Read the model definition and answer for the solid it produces. Units are mm, in the model's axes. A direction names the side the tool comes from. Coordinates: 2 decimals unless noted, no trailing zeros. Write each loop counter-clockwise with the first axis right and the second up, starting at its lowest first coordinate (ties: lowest second). Pieces come first, ordered by that corner, then holes.
(1) Which of the six approach directions +Z, -Z, +X, -X, +Y, -Y give full straight-line access (tool end or side, diameter ignored) to faces 1 (the flat face through (0, -50.5, -13)), 2 (the flat face through (0, -15, -13)), 3 (the cylindrical face through (-7.509, -2.535, 23.846))?
(2) Find the intervals of material crossed by probe 1 along X at (y, z) = (-60, 0) (3 decimals); probe 2 along Y at (x, z) = (22.5, 8.5); probe 3 along X at (y, z) = (-59, 11.5), in increasing order.
(3) Section C-C on x = -5.5 is taken. Write down the section's boundary in (y, z), then the cut area to 3 significant figures.
(4) Given pin 1 (5 mm diameter, centred on x = 0, z = -13.125, fed in from -Y); pin 2 (3 mm diameter, centred on x = 14, z = -0.5, fed in from +Y); pin 3 (8 mm diameter, centred on x = -5, y = -27.5, fed in from +Z), each flat-ended and moving along its own axis, determine where each tip first touches the part or whether it passes through.
(5) Section D-D on y = -39.5 is taken. Write down the section's boundary in (x, z).
(6) Section B-B on y = -58.5 is taken. Write down the section's boundary in (x, z) (3 decimals), then the cut area to 3 significant figures.
from build123d import *

# Parameters (mm, degrees)
SKIZZE5_R                       = 2.8
SCHNITT_LINEAR_AUSTRAGEN1_DEPTH = 15
SCHNITT_LINEAR_START            = -15
SKIZZE7_R                       = 2.8
SCHNITT_LINEAR_AUSTRAGEN2_DEPTH = 15


with BuildPart() as part:
    # Skizze4 → Rotation1 (revolve)
    with BuildSketch(Plane(origin=(0, 0, 0), x_dir=(0, 0, -1), z_dir=(1, 0, 0)), mode=Mode.PRIVATE) as rotation1_sk:
        Polygon((8.75, 0), (25, 0), (25, -5), (19.5, -5), (19.5, -6), (17.5, -6), (17.5, -65.5), (8.75, -65.5), align=None)
    revolve(rotation1_sk.sketch.rotate(Axis((0, 0, 0), (0, -1, 0)), 180), axis=Axis((0, 0, 0), (0, -1, 0)))

    # Skizze5 → Schnitt-Linear austragen1 (cut)
    with BuildSketch(Plane(origin=(0, 0, 0), x_dir=(1, 0, 0), z_dir=(0, 1, 0))):
        with Locations(Location((0, 13.125, 0), (0, 0, 270))):
            Circle(SKIZZE5_R)
        with Locations(Location((13.125, 0, 0), (0, 0, 270))):
            Circle(SKIZZE5_R)
        with Locations(Location((0, -13.125, 0), (0, 0, 270))):
            Circle(SKIZZE5_R)
        with Locations(Location((-13.125, 0, 0), (0, 0, 270))):
            Circle(SKIZZE5_R)
    extrude(amount=-SCHNITT_LINEAR_AUSTRAGEN1_DEPTH, mode=Mode.SUBTRACT)

    # Skizze7 → Schnitt-Linear austragen2 (cut)
    with BuildSketch(Plane.XZ.offset(65.5).offset(SCHNITT_LINEAR_START)):
        with Locations(Location((13.125, 0, 0), (0, 0, 90))):
            Circle(SKIZZE7_R)
        with Locations(Location((0, -13.125, 0), (0, 0, 90))):
            Circle(SKIZZE7_R)
        with Locations(Location((-13.125, 0, 0), (0, 0, 90))):
            Circle(SKIZZE7_R)
        with BuildLine():
            ThreePointArc((0, 15.925), (-2.8, 13.125), (0, 10.325))
            Line((0, 10.325), (0, 15.925))
        make_face()
        with BuildLine():
            Line((0, 15.925), (0, 10.325))
            ThreePointArc((0, 10.325), (1.979898987, 11.145101013), (2.8, 13.125))
            ThreePointArc((2.8, 13.125), (1.979898987, 15.104898987), (0, 15.925))
        make_face()
    extrude(amount=SCHNITT_LINEAR_AUSTRAGEN2_DEPTH, mode=Mode.SUBTRACT)


solid = part.part
Response:
1. face 1: -Y
1. face 2: +Y
1. face 3: +Y, -Y
2. probe 1: x = -17.5 to -15.925, -10.325 to -8.75, 8.75 to 10.325, 15.925 to 17.5
2. probe 2: y = -5 to 0
2. probe 3: x = -13.19 to -2.28, 2.28 to 13.19
3. outline: (-65.5, -16.61) - (-6, -16.61) - (-6, -18.71) - (-5, -18.71) - (-5, -24.39) - (0, -24.39) - (0, -6.81) - (-65.5, -6.81) - close; (-65.5, 6.81) - (0, 6.81) - (0, 24.39) - (-5, 24.39) - (-5, 18.71) - (-6, 18.71) - (-6, 16.61) - (-65.5, 16.61) - close
3. area: 1,370 mm2
4. pin 1: stops at y = -50.5
4. pin 2: stops at y = -15
4. pin 3: stops at z = 17.47
5. outline: circle Ø35 at (0, 0); hole circle Ø17.5 at (0, 0)
6. outline: circle Ø35 at (0, 0); hole circle Ø5.6 at (-13.125, 0); hole circle Ø17.5 at (0, 0); hole circle Ø5.6 at (0, -13.125); hole circle Ø5.6 at (0, 13.125); hole circle Ø5.6 at (13.125, 0)
6. area: 623 mm2
